Design review of the part built by this model. Coordinates are the model's own, in mm. Face numbers are marked on the shaded views. A direction names the side the tool comes from. Round coordinates to 2 decimals unless told otherwise and drop trailing zeros. Order: outer loops, then holes, each group sorted by start corner. A loop starts at its lowest first (then second) coordinate and runs counter-clockwise, first axis right, second up.
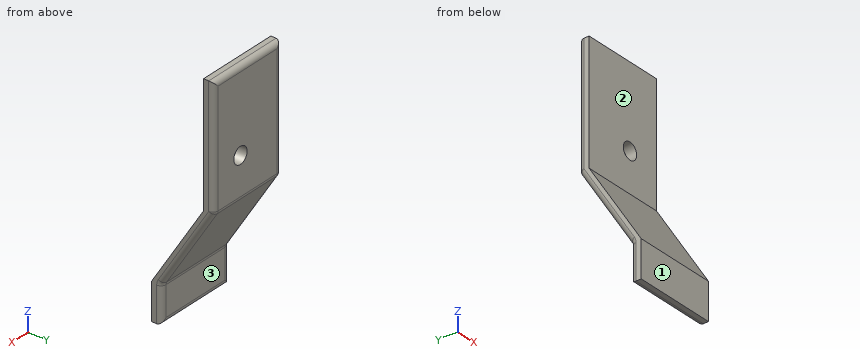
from build123d import *

# Parameters (mm, degrees)
SKETCH1_W           = 32
SKETCH1_H           = 92
BOSS_EXTRUDE1_DEPTH = 4
SKETCH2_R           = 3.175
CUT_EXTRUDE1_DEPTH  = 4
BOSS_EXTRUDE2_DEPTH = 32
CUT_EXTRUDE3_DEPTH  = 100.438423157
FILLET1_R           = 2


with BuildPart() as part:
    # Sketch1 → Boss-Extrude1 (new body)
    with BuildSketch(Plane(origin=(0, 0, 0), x_dir=(1, 0, 0), z_dir=(0, 1, 0))):
        with Locations((16, 46)):
            Rectangle(SKETCH1_W, SKETCH1_H)
    extrude(amount=BOSS_EXTRUDE1_DEPTH)

    # Sketch2 → Cut-Extrude1 (cut)
    with BuildSketch(Plane(origin=(0, 4, 0), x_dir=(1, 0, 0), z_dir=(0, 1, 0))):
        with Locations(Location((19.4, 31, 0), (0, 0, 270))):
            Circle(SKETCH2_R)
    extrude(amount=-CUT_EXTRUDE1_DEPTH, mode=Mode.SUBTRACT)

    # Sketch4 → Boss-Extrude2 (add)
    with BuildSketch(Plane(origin=(32, 0, 0), x_dir=(0, 0, -1), z_dir=(1, 0, 0))):
        Polygon((52.4, 0), (46, 0), (78, -20), (92, -20), (92, -16), (78, -16), align=None)
        Polygon((46, 4), (46, 0), (52.4, 0), align=None)
    extrude(amount=-BOSS_EXTRUDE2_DEPTH)

    # Sketch6 → Cut-Extrude3 (cut, through all)
    with BuildSketch(Plane(origin=(32, 0, 0), x_dir=(0, 0, -1), z_dir=(1, 0, 0))):
        Polygon((52.4, 0), (46, 4), (92, 4), (92, 0), align=None)
    extrude(amount=-CUT_EXTRUDE3_DEPTH, mode=Mode.SUBTRACT)

    # Fillet1
    fillet1_edges = [part.edges().sort_by_distance(p)[0] for p in [
        (32, 4, -23),
        (32, -16, -85),
        (16, -16, -78),
        (16, -16, -92),
        (32, -6, -62),
        (0, -6, -62),
        (0, -16, -85),
        (0, 4, -23),
        (16, 4, -46),
        (16, 4, 0),
    ]]
    fillet(fillet1_edges, radius=FILLET1_R)


solid = part.part
1) Take a section at B-B on z = -31. Give the boundary of the cut face in (x, y) (3 decimals), plus the area to 3 significant figures.
Results:
outline: (0, 0) - (16.225, 0) - (16.225, 4) - (2, 4) arc R2 ccw to (0, 2) - close; (22.575, 0) - (32, 0) - (32, 2) arc R2 ccw to (30, 4) - (22.575, 4) - close
area: 101 mm2
2) Clearance check with flat-ended pins moving along their axes: P1, Ø4, axis at x = 6, y = -2.5, coming from the +Z side; P2, Ø10, axis at x = 13, y = -8.5, coming from the -Z side; P3, Ø9, axis at x = 21, z = -87, coming from the +Y side. State where each tip first meets the part, or that it passes through.
Results:
P1: stops at z = -46.8
P2: stops at z = -74
P3: stops at y = -16
3) Take a section at C-C on x = 6.5. Give the boundary of the cut face in (y, z), plus the area to 3 significant figures.
Results:
outline: (-20, -92) - (-18, -92) arc R2 ccw to (-16, -90) - (-16, -78.57) arc R2 cw to (-15.7, -77.51) - (3.7, -46.49) arc R2 ccw to (4, -45.43) - (4, -2) arc R2 ccw to (2, 0) - (0, 0) - (0, -46) - (-20, -78) - close
area: 366 mm2
4) To check wall thickness, follow line 1 along X through (y, z) = (2.05, -31) (3 decimals); line 2 along Y through (x, z) = (29, -36); line 3 along Y through (x, z) = (21.5, -86). State the ranges of each line that lie inside material, in increasing order.
Results:
line 1: x = 0.001 to 16.225, 22.575 to 31.999
line 2: y = 0 to 4
line 3: y = -20 to -16
5) For the marked faces 1, 2 and 3, list the 3-axis set-ups (+Z, -Z, +X, -X, +Y, -Y) from which the entire face can be reached by the end or side of a thin tool; tool diameter is ignored.
Results:
face 1: +Z, -Z, +X, -X, -Y
face 2: +Z, +X, -X, -Y
face 3: -Z, +X, -X, +Y
6) Take a section at A-A on x = 19.4. Give the boundary of the cut face in (y, z) (3 decimals).
Results:
outline: (-20, -92) - (-18, -92) arc R2 ccw to (-16, -90) - (-16, -78.574) arc R2 cw to (-15.696, -77.514) - (3.696, -46.486) arc R2 ccw to (4, -45.426) - (4, -34.175) - (0, -34.175) - (0, -46) - (-20, -78) - close; (0, -27.825) - (4, -27.825) - (4, -2) arc R2 ccw to (2, 0) - (0, 0) - close
